```python
from build123d import *

# Parameters (mm, degrees)
SKETCH_W        = 44.5
SKETCH_H        = 22
SKETCH_R        = 1.75
SKETCH_R_2      = 1.25
PAD_DEPTH       = 4
SKETCH001_W     = 5.6
SKETCH001_H     = 5.6
POCKET_DEPTH    = 2
POCKET001_DEPTH = 2
SKETCH003_R     = 2.45
SKETCH003_R_2   = 1.25
PAD001_DEPTH    = 2
POCKET002_DEPTH = 4.001


with BuildPart() as part:
    # Sketch → Pad (new body)
    with BuildSketch(Plane.XY):
        Rectangle(SKETCH_W, SKETCH_H)
        with Locations((-12.5, 0)):
            Circle(SKETCH_R, mode=Mode.SUBTRACT)
        with Locations((12.5, 0)):
            Circle(SKETCH_R, mode=Mode.SUBTRACT)
        with Locations((-19.25, -8)):
            Circle(SKETCH_R_2, mode=Mode.SUBTRACT)
        with Locations((-5.75, 8)):
            Circle(SKETCH_R_2, mode=Mode.SUBTRACT)
        with Locations((19.25, 8)):
            Circle(SKETCH_R_2, mode=Mode.SUBTRACT)
        with Locations((5.75, -8)):
            Circle(SKETCH_R_2, mode=Mode.SUBTRACT)
    extrude(amount=PAD_DEPTH)

    # Sketch001 (on Face12 of Pad) → Pocket (cut)
    with BuildSketch(Plane.XY.offset(4)):
        with Locations((-12.5, 0)):
            Rectangle(SKETCH001_W, SKETCH001_H)
        with Locations((12.5, 0)):
            Rectangle(SKETCH001_W, SKETCH001_H)
    extrude(amount=-POCKET_DEPTH, mode=Mode.SUBTRACT)

    # Sketch002 → Pocket001 (cut)
    with BuildSketch(Plane(origin=(0, 0, 0), x_dir=(1, 0, 0), z_dir=(0, 0, -1))):
        Polygon((-3.7, -6.816432), (-5.75, -5.632864), (-7.8, -6.816432), (-7.8, -9.183568), (-5.75, -10.367136), (-3.7, -9.183568), align=None)
        Polygon((7.8, 9.183568), (5.75, 10.367136), (3.7, 9.183568), (3.7, 6.816432), (5.75, 5.632864), (7.8, 6.816432), align=None)
        Polygon((21.3, -6.816432), (19.25, -5.632864), (17.2, -6.816432), (17.2, -9.183568), (19.25, -10.367136), (21.3, -9.183568), align=None)
        Polygon((-17.2, 9.183568), (-19.25, 10.367136), (-21.3, 9.183568), (-21.3, 6.816432), (-19.25, 5.632864), (-17.2, 6.816432), align=None)
    extrude(amount=-POCKET001_DEPTH, mode=Mode.SUBTRACT)

    # Sketch003 (on Face5 of Pocket001) → Pad001 (join)
    with BuildSketch(Plane.XY.offset(4)):
        with Locations((-5.75, 8)):
            Circle(SKETCH003_R)
        with Locations((-5.75, 8)):
            Circle(SKETCH003_R_2, mode=Mode.SUBTRACT)
        with Locations((19.25, 8)):
            Circle(SKETCH003_R)
        with Locations((19.25, 8)):
            Circle(SKETCH003_R_2, mode=Mode.SUBTRACT)
        with Locations((5.75, -8)):
            Circle(SKETCH003_R)
        with Locations((5.75, -8)):
            Circle(SKETCH003_R_2, mode=Mode.SUBTRACT)
        with Locations((-19.25, -8)):
            Circle(SKETCH003_R)
        with Locations((-19.25, -8)):
            Circle(SKETCH003_R_2, mode=Mode.SUBTRACT)
    extrude(amount=PAD001_DEPTH)

    # Sketch004 (on Face5 of Pad001) → Pocket002 (cut, through all)
    with BuildSketch(Plane.XY.offset(4)):
        with BuildLine():
            Line((-21.05, 9.8), (-21.05, -3.875682))
            ThreePointArc((-17.7, -3.77537), (-19.384687, -3.502016), (-21.05, -3.875682))
            Line((-17.7, -3.77537), (-17.7, 5.2))
            Line((-17.7, 5.2), (-9.272783, 5.2))
            ThreePointArc((-9.874318, 9.8), (-10.212011, 7.41651), (-9.272783, 5.2))
            Line((-9.874318, 9.8), (-21.05, 9.8))
        make_face()
        with BuildLine():
            Line((17.7, 3.77537), (17.7, -5.2))
            Line((17.7, -5.2), (9.272783, -5.2))
            ThreePointArc((9.874318, -9.8), (10.212011, -7.41651), (9.272783, -5.2))
            Line((9.874318, -9.8), (21.05, -9.8))
            Line((21.05, -9.8), (21.05, 3.875682))
            ThreePointArc((17.7, 3.77537), (19.384687, 3.502016), (21.05, 3.875682))
        make_face()
        with BuildLine():
            Line((-7.3, 3.77537), (-7.3, 1.8))
            Line((-7.3, 1.8), (7.3, 1.8))
            Line((7.3, 1.8), (7.3, 5.2))
            Line((7.3, 5.2), (15.727217, 5.2))
            ThreePointArc((15.125682, 9.8), (14.787989, 7.41651), (15.727217, 5.2))
            Line((15.125682, 9.8), (-1.625682, 9.8))
            ThreePointArc((-7.3, 3.77537), (-2.474207, 4.914683), (-1.625682, 9.8))
        make_face()
        with BuildLine():
            Line((-7.3, -5.2), (-15.727217, -5.2))
            ThreePointArc((-15.125682, -9.8), (-14.787989, -7.41651), (-15.727217, -5.2))
            Line((-15.125682, -9.8), (1.625682, -9.8))
            ThreePointArc((7.3, -3.77537), (2.474207, -4.914683), (1.625682, -9.8))
            Line((7.3, -3.77537), (7.3, -1.8))
            Line((-7.3, -1.8), (7.3, -1.8))
            Line((-7.3, -1.8), (-7.3, -5.2))
        make_face()
    extrude(amount=-POCKET002_DEPTH, mode=Mode.SUBTRACT)


solid = part.part
```
The listing builds one solid part. Answer for the finished solid, in the listing's coordinates (mm). A direction names the side the tool comes from. Coordinates: 2 decimals unless noted, no trailing zeros. Write each loop counter-clockwise with the first axis right and the second up, starting at its lowest first coordinate (ties: lowest second). Pieces come first, ordered by that corner, then holes. Notation, with made-up numbers: (-18.75, 46) - (15.25, 46) arc R28 cw to (15.25, 84) - close; hole circle Ø3 at (72, 64). An arc over 180 degrees is marked (long way). Return JSON: item names as keys, results as strings. Group by question number.
Q1. The part is cut by section C-C on x = -12.5. Write down the section's boundary in (y, z), and give its area (3 significant figures).
Q2. Flat-ended cylindrical pins translate along their axes: pin 1 Ø2 at (x, y) = (-19.5, -9) entering from -Z; pin 2 Ø3 at (x, y) = (-12.5, 0) entering from -Z; pin 3 Ø3 at (x, y) = (11, 1) entering from +Z. Find the tip coordinate at first contact, or state that the pin passes through.
Q3. The part is cut by section A-A on z = 5.2. Write down the section's boundary in (x, y).
Q4. For a pull along X with two mould halves and no side action, classify faces 5 (the flat face through (-22.25, 0, 2)), 6 (the flat face through (6.789, -9.767, 0.986)), 7 (the flat face through (18, 9, 6)) as +X half, -X half, draft (parallel to the pull), parting line (faces both ways), or undercut.
Q5. Find the intervals of material crossed by line 1 along X through (y, z) = (0, 1); line 2 along X through (y, z) = (-8, 3); line 3 along Y through (x, z) = (-13, 3.9), in increasing order. Write a range as [from, to].
Q6. Which of the six approach directions +Z, -Z, +X, -X, +Y, -Y give full straight-line access (tool end or side, diameter ignored) to faces 1 (the flat face through (0, 11, 2)), 2 (the flat face through (-18.211, -9.767, 0.986)), 3 (the cylindrical face through (-3.413, 8.736, 4.986)), 4 (the flat face through (7, 9.8, 2))?
Q7. The part is cut by section B-B on y = 0. Write down the section's boundary in (x, z).
Q8. The part is cut by section D-D on z = 1.35. State how many separate pieces and enclosed holes the cut face has, and give its area (3 significant figures).
Evaluation:
{
 "1": {"outline": "(-11, 0) - (-9.8, 0) - (-9.8, 4) - (-11, 4) - close; (-5.2, 0) - (-1.75, 0) - (-1.75, 2) - (-2.8, 2) - (-2.8, 4) - (-5.2, 4) - close; (1.75, 0) - (5.2, 0) - (5.2, 4) - (2.8, 4) - (2.8, 2) - (1.75, 2) - close; (9.8, 0) - (11, 0) - (11, 4) - (9.8, 4) - close", "area": "33.0 mm2"},
 "2": {"pin 1": "stops at z = 2", "pin 2": "passes through", "pin 3": "stops at z = 4"},
 "3": {"outline": "circle Ø4.9 at (-19.25, -8); circle Ø4.9 at (-5.75, 8); circle Ø4.9 at (5.75, -8); circle Ø4.9 at (19.25, 8); hole circle Ø2.5 at (-19.25, -8); hole circle Ø2.5 at (-5.75, 8); hole circle Ø2.5 at (5.75, -8); hole circle Ø2.5 at (19.25, 8)"},
 "4": {"face 5": "-X half", "face 6": "undercut", "face 7": "draft"},
 "5": {"line 1": "x = [-22.25, -21.05], [-17.7, -14.25], [-10.75, 10.75], [14.25, 17.7], [21.05, 22.25]", "line 2": "x = [-22.25, -20.5], [-18, -14.75], [1.25, 4.5], [7, 10.25], [21.05, 22.25]", "line 3": "y = [-11, -9.8], [-5.2, -2.8], [2.8, 5.2], [9.8, 11]"},
 "6": {"face 1": "+Z, -Z, +X, -X, +Y", "face 2": "-Z", "face 3": "+Z", "face 4": "+Z, -Z"},
 "7": {"outline": "(-22.25, 0) - (-21.05, 0) - (-21.05, 4) - (-22.25, 4) - close; (-17.7, 0) - (-14.25, 0) - (-14.25, 2) - (-15.3, 2) - (-15.3, 4) - (-17.7, 4) - close; (-10.75, 0) - (10.75, 0) - (10.75, 2) - (9.7, 2) - (9.7, 4) - (-9.7, 4) - (-9.7, 2) - (-10.75, 2) - close; (14.25, 0) - (17.7, 0) - (17.7, 4) - (15.3, 4) - (15.3, 2) - (14.25, 2) - close; (21.05, 0) - (22.25, 0) - (22.25, 4) - (21.05, 4) - close"},
 "8": {"separate pieces": "1", "enclosed holes": "10", "area": "503 mm2"}
}
